Check sheet for the modelled part. Datum: model origin and axes. Units: mm. Round coordinates to 2 decimals unless told otherwise and drop trailing zeros. Write each loop counter-clockwise with the first axis right and the second up, starting at its lowest first coordinate (ties: lowest second). Pieces come first, ordered by that corner, then holes. Notation, with made-up numbers: M 28.25,82 L 75.25,82 A25 cw 75.25,118 Z; hole C -33,-14.75 d7. An arc over 180 degrees is marked long. Answer in a Markdown table with one row per item.
Autodesk Fusion 360 part; units mm, degrees
sketch "草图1" plane through (0, 0, 0) normal (0, 1, 0) x (1, 0, 0)
  line L0 (-14.7524, -4.7933) -> (-36.0595, 10.6872)
  circle A0 centre (0, 0) radius 40.6099
  line L1 (-5.9631, 12.5492) -> (0, 30.9017)
  line L2 (-9.1175, 12.5492) -> (-0.9789, 37.5972)
  line L3 (-35.4545, 12.5492) -> (-9.1175, 12.5492)
  line L4 (-29.3893, 9.5492) -> (-10.0923, 9.5492)
  line L5 (-13.7777, -1.7933) -> (-29.3893, 9.5492)
  line L6 (-18.1636, -25) -> (-12.2005, -6.6475)
  line L7 (-11.2257, -3.6475) -> (-6.9379, 9.5492)
  line L8 (-22.891, -29.8414) -> (-14.7524, -4.7933)
  line L9 (-13.7777, -1.7933) -> (-10.0923, 9.5492)
  line L10 (29.3893, 9.5492) -> (13.7777, -1.7933)
  line L11 (36.0595, 10.6872) -> (14.7524, -4.7933)
  line L12 (12.2005, -6.6475) -> (2.552, -13.6575)
  line L13 (0, -15.5116) -> (-21.3071, -30.9921)
  line L14 (18.1636, -25) -> (2.552, -13.6575)
  line L15 (0, -11.8034) -> (-11.2257, -3.6475)
  line L16 (21.3071, -30.9921) -> (0, -15.5116)
  line L17 (-2.552, -13.6575) -> (-12.2005, -6.6475)
  line L18 (11.2257, -3.6475) -> (0, -11.8034)
  line L19 (-2.552, -13.6575) -> (-18.1636, -25)
  line L20 (14.7524, -4.7933) -> (22.891, -29.8414)
  line L21 (0.9789, 37.5972) -> (9.1175, 12.5492)
  line L22 (10.0923, 9.5492) -> (13.7777, -1.7933)
  line L23 (0, 30.9017) -> (5.9631, 12.5492)
  line L24 (-6.9379, 9.5492) -> (6.9379, 9.5492)
  line L25 (10.0923, 9.5492) -> (29.3893, 9.5492)
  line L26 (-5.9631, 12.5492) -> (5.9631, 12.5492)
  line L27 (9.1175, 12.5492) -> (35.4545, 12.5492)
  line L28 (6.9379, 9.5492) -> (11.2257, -3.6475)
  line L29 (12.2005, -6.6475) -> (18.1636, -25)
  arc A1 (-0.9789, 37.5972) -> (-35.4545, 12.5492) centre (0, 0) ccw
  arc A2 (35.4545, 12.5492) -> (0.9789, 37.5972) centre (0, 0) ccw
  arc A3 (22.891, -29.8414) -> (36.0595, 10.6872) centre (0, 0) ccw
  arc A4 (-36.0595, 10.6872) -> (-22.891, -29.8414) centre (0, 0) ccw
  arc A5 (-21.3071, -30.9921) -> (21.3071, -30.9921) centre (0, 0) ccw
extrude "拉伸1" add sketch "草图1" along normal blind 5 makes body 1
sketch "草图2" plane through (0, 5, 0) normal (0, 1, 0) x (-1, 0, 0)
  arc A0 (21.3071, 30.9921) -> (-21.3071, 30.9921) centre (0, 0) ccw
  line L0 (21.3071, 30.9921) -> (0, 15.5116)
  line L1 (0, 15.5116) -> (-21.3071, 30.9921)
  arc A1 (-22.891, 29.8414) -> (-36.0595, -10.6872) centre (0, 0) ccw
  line L2 (-22.891, 29.8414) -> (-14.7524, 4.7933)
  line L3 (-14.7524, 4.7933) -> (-36.0595, -10.6872)
  arc A2 (-35.4545, -12.5492) -> (-0.9789, -37.5972) centre (0, 0) ccw
  line L4 (-35.4545, -12.5492) -> (-9.1175, -12.5492)
  line L5 (-9.1175, -12.5492) -> (-0.9789, -37.5972)
  arc A3 (36.0595, -10.6872) -> (22.891, 29.8414) centre (0, 0) ccw
  line L6 (36.0595, -10.6872) -> (14.7524, 4.7933)
  line L7 (14.7524, 4.7933) -> (22.891, 29.8414)
  line L8 (6.9379, -9.5492) -> (-6.9379, -9.5492)
  line L9 (-6.9379, -9.5492) -> (-11.2257, 3.6475)
  line L10 (-11.2257, 3.6475) -> (0, 11.8034)
  line L11 (0, 11.8034) -> (11.2257, 3.6475)
  line L12 (11.2257, 3.6475) -> (6.9379, -9.5492)
  line L13 (-2.552, 13.6575) -> (-12.2005, 6.6475)
  line L14 (-12.2005, 6.6475) -> (-18.1636, 25)
  line L15 (-18.1636, 25) -> (-2.552, 13.6575)
  arc A4 (0.9789, -37.5972) -> (35.4545, -12.5492) centre (0, 0) ccw
  line L16 (0.9789, -37.5972) -> (9.1175, -12.5492)
  line L17 (9.1175, -12.5492) -> (35.4545, -12.5492)
  line L18 (5.9631, -12.5492) -> (0, -30.9017)
  line L19 (0, -30.9017) -> (-5.9631, -12.5492)
  line L20 (-5.9631, -12.5492) -> (5.9631, -12.5492)
  line L21 (-13.7777, 1.7933) -> (-10.0923, -9.5492)
  line L22 (-10.0923, -9.5492) -> (-29.3893, -9.5492)
  line L23 (-29.3893, -9.5492) -> (-13.7777, 1.7933)
  line L24 (12.2005, 6.6475) -> (2.552, 13.6575)
  line L25 (2.552, 13.6575) -> (18.1636, 25)
  line L26 (18.1636, 25) -> (12.2005, 6.6475)
  line L27 (13.7777, 1.7933) -> (29.3893, -9.5492)
  line L28 (29.3893, -9.5492) -> (10.0923, -9.5492)
  line L29 (10.0923, -9.5492) -> (13.7777, 1.7933)
  circle A5 centre (0, 0) radius 40.6099
  circle A6 centre (55, 0) radius 2.5
  circle A7 centre (55, 0) radius 4
  dimension "d5" = 8
extrude "拉伸2" add sketch "草图2" along normal blind 5 separate body contours A7 makes body 2
move_body "移动1" bodies 2 to x (1, 0, 0) y (0, 1, 0) z (0, 0, 1) at (0, -5, 0)
move_body "移动2" bodies 2 to x (1, 0, 0) y (0, 1, 0) z (0, 0, 1) at (55.2046, 0, -43.1842)
combine "合并1" operation add target body 1 tool bodies 2
1. Scan lines: L1, parallel to X at y = 4, z = -32; L2, parallel to X at y = 0.6, z = 17.5; L3, parallel to X at y = 4.75, z = -15. Record each from-to range of solid material in increasing order.
Found:
| item | result |
|---|---|
| L1 | x = -25 to -19.76, -2.8 to 2.8, 19.76 to 25 |
| L2 | x = -36.65 to -33.29, -18.88 to -15.73, -7.84 to -2.74, 2.74 to 7.84, 15.73 to 18.88, 33.29 to 36.65 |
| L3 | x = -37.74 to -34.49, -8.32 to -5.17, 5.17 to 8.32, 34.49 to 37.74 |
2. Section check A-A, the plane z = -18. Record the cut outline in (x, y).
Found:
| item | result |
|---|---|
| outline | M -36.4,0 L -33.02,0 L -33.02,5 L -36.4,5 Z; M -7.35,0 L -4.19,0 L -4.19,5 L -7.35,5 Z; M 4.19,0 L 7.35,0 L 7.35,5 L 4.19,5 Z; M 33.02,0 L 36.4,0 L 36.4,5 L 33.02,5 Z |
3. Section check C-C, the plane z = -4. Record the cut outline in (x, y).
Found:
| item | result |
|---|---|
| outline | M -40.41,0 L -37.4,0 L -37.4,5 L -40.41,5 Z; M -26.86,0 L -21.75,0 L -21.75,5 L -26.86,5 Z; M -11.9,0 L -8.74,0 L -8.74,5 L -11.9,5 Z; M 8.74,0 L 11.9,0 L 11.9,5 L 8.74,5 Z; M 21.75,0 L 26.86,0 L 26.86,5 L 21.75,5 Z; M 37.4,0 L 40.41,0 L 40.41,5 L 37.4,5 Z |
4. Section check B-B, the plane x = -31.5. Record the cut outline in (y, z).
Found:
| item | result |
|---|---|
| outline | M 0,-25.63 L 5,-25.63 L 5,-20.55 L 0,-20.55 Z; M 0,-12.55 L 5,-12.55 L 5,-7.37 L 0,-7.37 Z; M 0,20.55 L 5,20.55 L 5,25.63 L 0,25.63 Z |
5. Section check D-D, the plane z = -28. Record the cut outline in (x, y), and give its area (3 significant figures).
Found:
| item | result |
|---|---|
| outline | M -29.41,0 L -25.11,0 L -25.11,5 L -29.41,5 Z; M -4.1,0 L -0.94,0 L -0.94,5 L -4.1,5 Z; M 0.94,0 L 4.1,0 L 4.1,5 L 0.94,5 Z; M 25.11,0 L 29.41,0 L 29.41,5 L 25.11,5 Z |
| area | 74.6 mm2 |
6. Go/stop test with flat-tipped pins: pin 1 (4 mm diameter, centred on x = 0.2, z = -43.18, fed in from -Y); pin 2 (2.5 mm diameter, centred on x = -2.5, y = 2.5, fed in from +Z); pin 3 (1.5 mm diameter, centred on x = -16.5, y = 3.5, fed in from +Z); pin 4 (1 mm diameter, centred on y = 2.5, z = 4, fed in from +X). Record where each tip stops, or that it passes through.
Found:
| item | result |
|---|---|
| pin 1 | passes through |
| pin 2 | stops at z = 40.59 |
| pin 3 | stops at z = 37.43 |
| pin 4 | stops at x = 40.46 |
7. Draft check along X on faces 1 (the face through (-9, 5, -7)), 2 (the face through (21.693, 2.465, -3.957)). Enter one of: +X half, -X half, draft (parallel to the pull), parting line (faces both ways), or undercut.
Found:
| item | result |
|---|---|
| face 1 | draft |
| face 2 | undercut |
